Geometry: see drawing. Coordinates: mm, zero at the bounding-box minimum. Give positions to 0.01 mm unless a question says otherwise; leave off trailing zeros. Loops run counter-clockwise (first coordinate to the right, second up) from the corner with the lowest first, then second, coordinate; pieces in that order, holes last. Notation, with made-up numbers: (45.5, -23) -> (82.5, -23) arc R27 cw to (82.5, 16) -> close; hole circle Ø5 at (-30.75, 63.25). An arc over 180 degrees is marked (long way). Use CSV: the item, a comma, the result in double quotes.
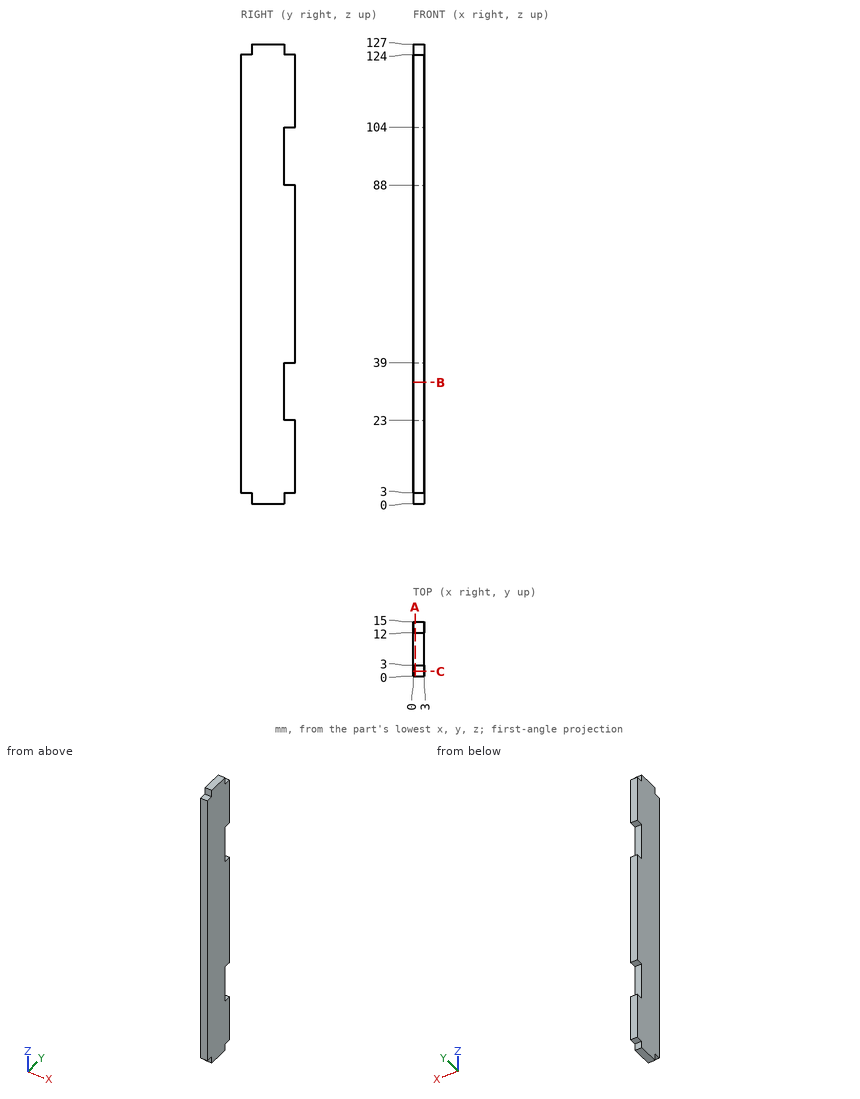
1) Section query C-C (y = 1.25). Return loops of the section in (x, z).
From the geometry:
outline,"(0, 3) -> (3, 3) -> (3, 124) -> (0, 124) -> close"
2) Section query B-B (z = 33.5). Return loops of the section in (x, y).
From the geometry:
outline,"(0, 0) -> (3, 0) -> (3, 12) -> (0, 12) -> close"
3) Ray query, line 1 (Z direction, x = 2, y = 12.75); line 2 (Y direction, x = 1.2, z = 92.5). Return the intervals inside material, ascending.
From the geometry:
line 1,"z = 3 to 23, 39 to 88, 104 to 124"
line 2,"y = 0 to 12"
4) Section query A-A (x = 0.55). Return loops of the section in (y, z).
From the geometry:
outline,"(0, 3) -> (3, 3) -> (3, 0) -> (12, 0) -> (12, 3) -> (15, 3) -> (15, 23) -> (12, 23) -> (12, 39) -> (15, 39) -> (15, 88) -> (12, 88) -> (12, 104) -> (15, 104) -> (15, 124) -> (12, 124) -> (12, 127) -> (3, 127) -> (3, 124) -> (0, 124) -> close"
5) Contact query for flat-ended pins moving along their axis: pin 1 (0.9 mm diameter, centred on x = 1, z = 1, fed in from -Y); pin 2 (0.9 mm diameter, centred on x = 1, y = 2, fed in from +Z); pin 3 (1.5 mm diameter, centred on x = 2, z = 29.5, fed in from +Y). Output: stop coordinate, or through.
From the geometry:
pin 1,"stops at y = 3"
pin 2,"stops at z = 124"
pin 3,"stops at y = 12"
